Study the drawing (mm; zero at the part's minimum x, y, z) and answer. A direction names the side the tool comes from. Coordinates: 2 decimals unless noted, no trailing zeros. Order: outer loops, then holes, each group sorted by start corner. A loop starts at its lowest first (then second) coordinate and runs counter-clockwise, first axis right, second up.
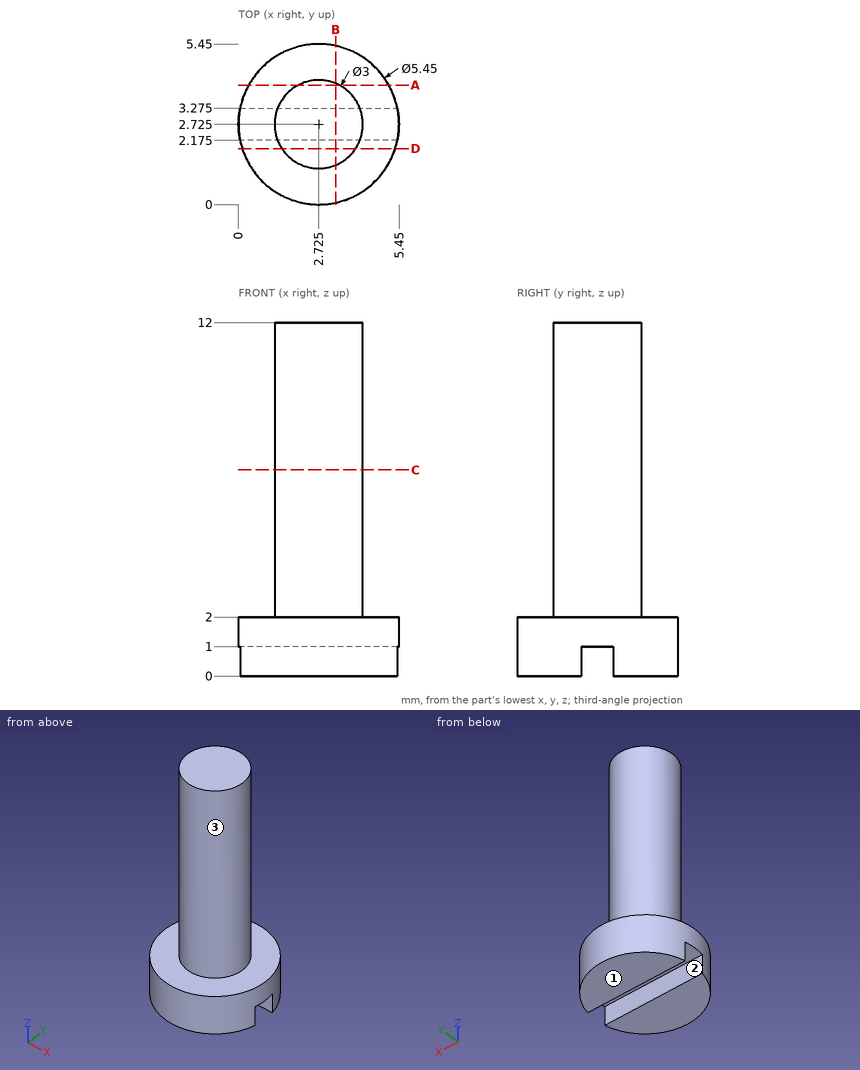
1) A cutting plane is placed at D-D, the plane y = 1.9. Determine the outline of the cut face in (x, z).
A:
outline: (0.13, 0) - (5.32, 0) - (5.32, 2) - (3.98, 2) - (3.98, 12) - (1.47, 12) - (1.47, 2) - (0.13, 2) - close
2) Straight lines are drawn through the part: line 1 (Z direction, x = 4.8, y = 1.75); line 2 (Y direction, x = 2.7, z = 7.5); line 3 (Z direction, x = 5, y = 2.85). For each, find the intervals that lie inside material, in ascending order.
A:
line 1: z = 0 to 2
line 2: y = 1.23 to 4.22
line 3: z = 1 to 2
3) Which of the six approach directions +Z, -Z, +X, -X, +Y, -Y give full straight-line access (tool end or side, diameter ignored) to the marked faces 1, 2 and 3?
A:
face 1: -Z, +X, -X, +Y, -Y
face 2: -Z, +X, -X
face 3: +Z
4) Flat-ended cylindrical pins translate along their axes: pin 1 Ø0.5 at (x, z) = (1.5, 0.5) entering from -Y; pin 2 Ø1.5 at (y, z) = (3.5, 6) entering from +X; pin 3 Ø1 at (x, z) = (3, 3.5) entering from -Y (3 decimals). Find the tip coordinate at first contact, or state that the pin passes through.
A:
pin 1: stops at y = 0.18
pin 2: stops at x = 4.22
pin 3: stops at y = 1.225
5) A cutting plane is placed at B-B, the plane x = 3.3. Determine the outline of the cut face in (y, z) (3 decimals).
A:
outline: (0.061, 0) - (2.175, 0) - (2.175, 1) - (3.275, 1) - (3.275, 0) - (5.389, 0) - (5.389, 2) - (4.11, 2) - (4.11, 12) - (1.34, 12) - (1.34, 2) - (0.061, 2) - close
6) A cutting plane is placed at C-C, the plane z = 7. Determine the outline of the cut face in (x, y) (3 decimals).
A:
outline: circle Ø3 at (2.725, 2.725)
7) A cutting plane is placed at A-A, the plane y = 4.05. Determine the outline of the cut face in (x, z).
A:
outline: (0.34, 0) - (5.11, 0) - (5.11, 2) - (3.43, 2) - (3.43, 12) - (2.02, 12) - (2.02, 2) - (0.34, 2) - close
